Read the model definition and answer for the solid it produces. Units are mm, in the model's axes. A direction names the side the tool comes from. Give positions to 0.01 mm unless a question says otherwise; leave off trailing zeros. Loops run counter-clockwise (first coordinate to the right, second up) from the corner with the lowest first, then second, coordinate; pieces in that order, holes last. Notation, with made-up numbers: (52.5, 61.5) -> (85.5, 61.5) arc R28 ccw to (85.5, 92.5) -> close; hole circle Ø4 at (-8.75, 4.25). An arc over 180 degrees is marked (long way). One line per item, written item: value. Start each with the question number.
from build123d import *

# Parameters (mm, degrees)
SKETCH5_W           = 12.880016042
SKETCH5_H           = 15.834691301
CUT_EXTRUDE2_DEPTH  = 7.62
BOSS_EXTRUDE1_DEPTH = 3.175
CUT_EXTRUDE4_DEPTH  = 1.5875
SKETCH10_W          = 4
SKETCH10_H          = 3.30542238
CUT_EXTRUDE5_DEPTH  = 34.174999944


with BuildPart() as part:
    # Sketch2 → Revolve1 (revolve)
    with BuildSketch(Plane(origin=(0, 0, 0), x_dir=(0, 0, -1), z_dir=(1, 0, 0))):
        Polygon((0, -50.8), (-29.999999944, 0), (0, 0), align=None)
    revolve(axis=Axis((0, 0, 0), (0, -1, 0)))

    # Sketch4 → Cut-Revolve1 (revolve, cut)
    with BuildSketch(Plane(origin=(0, 0, 0), x_dir=(0, 0, -1), z_dir=(1, 0, 0))):
        Polygon((0, -45.72), (-24.919999944, 0), (0, 0), align=None)
    revolve(axis=Axis((0, 16.11457811, 0), (0, -1, 0)), mode=Mode.SUBTRACT)

    # Sketch5 → Cut-Extrude2 (cut, symmetric)
    with BuildSketch(Plane(origin=(0, 0, 0), x_dir=(0, 0, -1), z_dir=(1, 0, 0))):
        with Locations((0, -47.812265381)):
            Rectangle(SKETCH5_W, SKETCH5_H)
    extrude(amount=CUT_EXTRUDE2_DEPTH, both=True, mode=Mode.SUBTRACT)

    # Sketch6 → Boss-Extrude1 (add, symmetric)
    with BuildSketch(Plane(origin=(0, 0, 0), x_dir=(0, 0, -1), z_dir=(1, 0, 0))):
        with BuildLine():
            Line((0, -39.89491973), (-7.374618631, -39.89491973))
            Line((-7.374618631, -39.89491973), (8.649316149, -67.028782674))
            ThreePointArc((8.649316149, -67.028782674), (24.995151659, -85.745993658), (46.99, -97.31089625))
            ThreePointArc((46.99, -97.31089625), (56.876704451, -99.570972509), (66.99, -100.33))
            Line((66.99, -100.33), (70.165, -100.33))
            Line((70.165, -100.33), (70.165, -90.805))
            Line((70.165, -90.805), (66.99, -90.805))
            Line((66.99, -90.805), (66.99, -93.98))
            ThreePointArc((66.99, -93.98), (36.549925695, -85.903846215), (14.117056519, -63.799802147))
            Line((14.117056519, -63.799802147), (0, -39.89491973))
        make_face()
        Polygon((-30.934610553, 0), (-7.374618631, -39.89491973), (0, -39.89491973), (-23.559991923, 0), align=None)
    extrude(amount=BOSS_EXTRUDE1_DEPTH, both=True)

    # Sketch7 → Cut-Extrude4 (cut)
    with BuildSketch(Plane(origin=(0, 0, 0), x_dir=(0, 0, -1), z_dir=(1, 0, 0))):
        with BuildLine():
            Line((-3.175, -39.89491973), (11.763026223, -65.189977515))
            ThreePointArc((11.763026223, -65.189977515), (31.846754922, -86.228834252), (59.157727955, -96.233853156))
            ThreePointArc((59.157727955, -96.233853156), (63.072632016, -96.704901626), (66.99, -97.155))
            Line((66.99, -97.155), (66.99, -93.98))
            ThreePointArc((66.99, -93.98), (58.670725699, -93.413828019), (50.504865217, -91.725752721))
            ThreePointArc((50.504865217, -91.725752721), (29.605505433, -81.288014454), (14.117056519, -63.799802147))
            Line((14.117056519, -63.799802147), (-23.559991923, 0))
            Line((-23.559991923, 0), (-26.734991923, 0))
            Line((-26.734991923, 0), (-3.175, -39.89491973))
        make_face()
    cut_extrude4 = extrude(amount=-CUT_EXTRUDE4_DEPTH, mode=Mode.SUBTRACT)

    # Mirror1: Cut-Extrude4 across plane
    add(cut_extrude4.mirror(Plane(origin=(0, 0, 0), x_dir=(0, 0, 1), z_dir=(1, 0, 0))), mode=Mode.SUBTRACT)

    # Sketch9 → Cut-Revolve2 (revolve, cut)
    with BuildSketch(Plane(origin=(0, 0, 0), x_dir=(0, 0, -1), z_dir=(1, 0, 0))):
        Polygon((0, 0), (-24.9199908, 0), (-2.801476321, -39.89491973), (0, -39.89491973), align=None)
    revolve(axis=Axis((0, 16.11457811, 0), (0, -1, 0)), mode=Mode.SUBTRACT)

    # Sketch10 → Cut-Extrude5 (cut, through all)
    with BuildSketch(Plane.ZY.offset(3.175)):
        with Locations((-64.99, -95.50228881)):
            Rectangle(SKETCH10_W, SKETCH10_H)
    extrude(amount=-CUT_EXTRUDE5_DEPTH, mode=Mode.SUBTRACT)


solid = part.part
Item 1: Section C-C, the plane z = -40 is taken. Determine the outline of the cut face in (x, y) (1 decimal).
Item 2: Section A-A, the plane x = 0 is taken. Determine the outline of the cut face in (y, z) (1 decimal), plus the area to 3 significant figures.
Item 3: Flat-ended cylindrical pins translate along their axes: pin 1 (9.5 mm diameter, centred on x = 0.5, z = -2, fed in from -Y); pin 2 (20 mm diameter, centred on y = -12.5, z = 7, fed in from -X); pin 3 (1 mm diameter, centred on x = -2, z = 0.5, fed in from +Y). Find the tip coordinate at first contact, or state that the pin passes through.
Item 4: Determine the mould class of faces 4 (the flat face through (0, -97.155, -65)), 5 (the flat face through (1.588, -70, -18)), 6 (the cylindrical face through (2.39, -85.1, -35.18)), 7 (the flat face through (0, -100.33, -69)) for opening direction Y: pulls with the +Y half, pulls with the -Y half, needs draft (parallel to the pull), parting line crosses it, or undercut.
Item 5: Consider L1, parallel to X at y = -92, z = -45 (1 decimal); L2, parallel to Z at x = -5.5, y = -32; L3, parallel to Z at x = -8, y = -6.5. Determine where each line is inside the solid, lowest interval first. Write a range as [from, to].
Item 6: For faces 1 (the cylindrical face through (-2.37, -85.1, -35.18)), 2 (the conical face through (2.309, -28.906, 8.589)), 3 (the flat face through (2, -39.895, -3)), determine the directions among +Z, -Z, +X, -X, +Y, -Y from which every point of the face is accessible in a straight line to the end or side of a thin tool.
Item 7: Section D-D, the plane y = -80.5 is taken. Determine the outline of the cut face in (x, z) (1 decimal).
Computed values:
1. outline: (-3.2, -94.7) -> (3.2, -94.7) -> (3.2, -87.7) -> (1.6, -87.7) -> (1.6, -90.8) -> (-1.6, -90.8) -> (-1.6, -87.7) -> (-3.2, -87.7) -> close
2. outline: (-100.3, -70.2) -> (-90.8, -70.2) -> (-90.8, -67) -> (-97.2, -67) -> (-97.2, -63) -> (-96.7, -63) arc R737.1 cw to (-96.2, -59.2) arc R64.1 cw to (-65.2, -11.8) -> (0, 26.7) -> (0, 30.9) -> (-67, -8.6) arc R67.8 ccw to (-100.3, -67) -> close; (-39.9, -6.4) -> (0, -30) -> (0, -24.9) -> (-39.9, -3.2) -> close
2. area: 720 mm²
3. pin 1: y = -63.81
3. pin 2: x = -27.98
3. pin 3: y = -39.89
4. face 4: pulls with the +Y half
4. face 5: undercut
4. face 6: undercut
4. face 7: pulls with the -Y half
5. L1: [-3.2, -1.6], [1.6, 3.2]
5. L2: [-9.64, -5.07], [5.07, 9.64]
5. L3: [-24.91, -19.82], [19.82, 24.91]
6. face 1: +X, -X
6. face 2: +Y
6. face 3: -Z
7. outline: (-3.2, -28.6) -> (-1.6, -28.6) -> (-1.6, -24.4) -> (1.6, -24.4) -> (1.6, -28.6) -> (3.2, -28.6) -> (3.2, -19.1) -> (-3.2, -19.1) -> close
